```python
from build123d import *

# Parameters (mm, degrees)
F0_R      = 44.45
F1_DEPTH  = 12.7
F2_R      = 41.275
F3_DEPTH  = 12.7
F4_R      = 41.275
F5_DEPTH  = 9.525
F7_R      = 2.833981
F8_DEPTH  = 57.15
F11_R     = 1.713895
F12_DEPTH = 57.15
F6_R      = 36.5125
F15_DEPTH = 12.7


with BuildPart() as f1:
    # F0 (on Top) → F1 (new body, symmetric)
    with BuildSketch(Plane.XY):
        Circle(F0_R)
    extrude(amount=F1_DEPTH, both=True)

    # F2 (on Top) → F3 (cut, symmetric)
    with BuildSketch(Plane.XY):
        Circle(F2_R)
    extrude(amount=F3_DEPTH, both=True, mode=Mode.SUBTRACT)

    # F4 (on Top) → F5 (join, symmetric)
    with BuildSketch(Plane.XY):
        Circle(F4_R)
    extrude(amount=F5_DEPTH, both=True)

    # F7 (on Front) → F8 (join, symmetric)
    with BuildSketch(Plane.XZ):
        Circle(F7_R)
    extrude(amount=F8_DEPTH, both=True)

    # F9 (on Right) → F10 (revolve)
    with BuildSketch(Plane.YZ):
        Polygon((-51.933423, -2.833975), (-55.044275, -2.833975), (-51.933423, -3.468975), align=None)
    revolve(axis=Axis((0, -57.15, 0), (0, -1, 0)))

    # F11 (on Front) → F12 (cut, symmetric)
    with BuildSketch(Plane.XZ):
        Circle(F11_R)
    extrude(amount=F12_DEPTH, both=True, mode=Mode.SUBTRACT)

    # F13 (on Right) → F14 (revolve)
    with BuildSketch(Plane.YZ):
        Polygon((51.421318, -3.514614), (54.515656, -2.803493), (51.421318, -2.874012), align=None)
    revolve(axis=Axis((0, 57.15, 0), (0, -1, 0)))

    # F6 (on Top) → F15 (cut, symmetric)
    with BuildSketch(Plane.XY):
        Circle(F6_R)
    extrude(amount=F15_DEPTH, both=True, mode=Mode.SUBTRACT)


solid = f1.part
```
Here's how the part is built. I have some questions about the finished solid (model axes, mm). A direction names the side the tool comes from. Round coordinates to 2 decimals unless told otherwise and drop trailing zeros. Order: outer loops, then holes, each group sorted by start corner. A loop starts at its lowest first (then second) coordinate and runs counter-clockwise, first axis right, second up. Notation, with made-up numbers: M 88,27.25 L 138,27.25 A36 ccw 138,61.25 Z; hole C 42.5,0.25 d4. An arc over 180 degrees is marked long. Answer as CSV lines item,"result".
Item 1: For pin 1 (1 mm diameter, centred on x = -10, z = 6, fed in from +Y); pin 2 (8 mm diameter, centred on y = 31, z = -2, fed in from +X); pin 3 (5 mm diameter, centred on y = -33.5, z = -4, fed in from -X), each with a flat end and sliding along its axis, tell me the tip position at first contact or that it passes through.
From the geometry:
pin 1,"y = 43.42"
pin 2,"x = 35.31"
pin 3,"x = -31.86"
Item 2: Imagine slicing it at C-C on x = -24.5. List the corners of the cut face in (y, z) for me (3 decimals), and give its area (3 significant figures).
From the geometry:
outline,"M -37.088,-12.7 L -33.217,-12.7 L -33.217,-9.525 L -27.072,-9.525 L -27.072,9.525 L -33.217,9.525 L -33.217,12.7 L -37.088,12.7 Z; M 27.072,-9.525 L 33.217,-9.525 L 33.217,-12.7 L 37.088,-12.7 L 37.088,12.7 L 33.217,12.7 L 33.217,9.525 L 27.072,9.525 Z"
area,"431 mm2"
Item 3: Please list where these lines run through material, in increasing order: L1, parallel to Y at x = 0, z = -11.15 (3 decimals); L2, parallel to X at y = 44.75, z = 0; L3, parallel to Y at x = 0, z = 5.75. Write a range as [from, to].
From the geometry:
L1,"[-44.45, -41.275], [41.275, 44.45]"
L2,"[-2.83, -1.71], [1.71, 2.83]"
L3,"[-44.45, -36.51], [36.51, 44.45]"
Item 4: Which directions (+Z, -Z, +X, -X, +Y, -Y) give clear straight access to the entire face, cutting with the end or side of a thin tool? Please do faces 1 (the flat face through (15.09, -33.44, 9.525)), 2 (the cylindrical face through (-0.37, -56.11, 2.81)), 3 (the cylindrical face through (-0.614, -48.2, -2.767)), 4 (the flat face through (15.09, -33.44, -9.525)), 5 (the cylindrical face through (-0.37, 55.75, 2.81)).
From the geometry:
face 1,"+Z"
face 2,"-Y"
face 3,"none"
face 4,"-Z"
face 5,"+Y"
Item 5: Imagine slicing it at D-D on x = 0. Give the number of separate pieces and of enclosed holes in the cut face, and give its area (3 significant figures).
From the geometry:
separate pieces,"4"
enclosed holes,"0"
area,"349 mm2"
Item 6: We'd pull the mould along Y, two halves only. Please class faces 6 (the flat face through (29.4, -29.4, 12.7)), 7 (the cylindrical face through (-8.948, -40.293, 11.135)), 8 (the conical face through (-2.947, 53.581, 0.654)): +Y half, -Y half, draft (parallel to the pull), parting line (faces both ways), or undercut.
From the geometry:
face 6,"draft"
face 7,"undercut"
face 8,"+Y half"
